Geometry check sheet. Reference: the model listing, model coordinates, mm. Coordinates: 2 decimals unless noted, no trailing zeros. Order: outer loops, then holes, each group sorted by start corner. A loop starts at its lowest first (then second) coordinate and runs counter-clockwise, first axis right, second up. Notation, with made-up numbers: M 69,-22.75 L 97,-22.75 A10 ccw 97,-8.75 Z; hole C 75,-39 d6. An arc over 180 degrees is marked long. One line per item, written item: value. Start each with the question number.
1) Sectioned sample at A-A, the plane x = 26. Enter the section's corners in (y, z) (3 decimals).
2) Sectioned sample at D-D, the plane x = 145. Enter the section's corners in (y, z) (3 decimals).
3) Sectioned sample at C-C, the plane y = 1.75. State how many separate pieces and enclosed holes the cut face has, then the cut area to 3 significant figures.
4) Thickness scan on L1, parallel to Z at x = 151, y = 2.2; L2, parallel to Z at x = 104.5, y = 0.5 (3 decimals); L3, parallel to X at y = 3, z = -44. Record the ranges inside material, lowest first. Write a range as from..to.
5) Go/stop test with a flat-tipped pin: P1, Ø2.5, axis at x = 4, z = -4, coming from the +Y side. Record where the tip stops, or that it passes through.
6) Draft check along X on faces 1 (the flat face through (0, 1, -35)), 2 (the flat face through (82, 0, -25)), 3 (the flat face through (155, 1, -35)). Enter one of: pulls with the +X half, pulls with the -X half, needs draft (parallel to the pull), parting line crosses it, or undercut.
```python
from build123d import *

# Parameters (mm, degrees)
SKETCH1_R           = 1.5
SKETCH1_W           = 19.05
SKETCH1_H           = 19.05
BOSS_EXTRUDE1_DEPTH = 3.75
SKETCH2_W           = 9.525
SKETCH2_H           = 3.75
BOSS_EXTRUDE2_DEPTH = 20
SKETCH3_W           = 17.05
SKETCH3_H           = 3.75
CUT_EXTRUDE1_DEPTH  = 2
SKETCH4_W           = 88.15
SKETCH4_H           = 3.75
BOSS_EXTRUDE3_DEPTH = 4
SKETCH5_W           = 13.325
SKETCH5_H           = 3.75
BOSS_EXTRUDE4_DEPTH = 6
SKETCH6_W           = 19.675
SKETCH6_H           = 3.75
BOSS_EXTRUDE5_DEPTH = 10
SKETCH7_W           = 11
SKETCH7_H           = 3.75
CUT_EXTRUDE2_DEPTH  = 4
SKETCH8_W           = 33
SKETCH8_H           = 3.75
BOSS_EXTRUDE6_DEPTH = 1.0375
SKETCH9_W           = 38.1
SKETCH9_H           = 3.75
CUT_EXTRUDE3_DEPTH  = 0.5
SKETCH10_W          = 52.725
SKETCH10_H          = 3.75
CUT_EXTRUDE4_DEPTH  = 0.5
SKETCH11_W          = 18
SKETCH11_H          = 3.75
CUT_EXTRUDE5_DEPTH  = 0.5
SKETCH13_W          = 14.7
SKETCH13_H          = 3.75
CUT_EXTRUDE6_DEPTH  = 2.175
FILLET1_R           = 0.5
BOSS_EXTRUDE7_START = 3
BOSS_EXTRUDE7_DEPTH = 3
FILLET2_R           = 0.5
FILLET3_R           = 0.5


with BuildPart() as part:
    # Sketch1 → Boss-Extrude1 (new body)
    with BuildSketch(Plane(origin=(0, 0, 0), x_dir=(1, 0, 0), z_dir=(0, 1, 0))):
        with BuildLine():
            ThreePointArc((0, 0.5), (0.146446609, 0.146446609), (0.5, 0))
            Line((0.5, 0), (154.5, 0))
            ThreePointArc((154.5, 0), (154.853553391, 0.146446609), (155, 0.5))
            Line((155, 0.5), (155, 69.5))
            ThreePointArc((155, 69.5), (154.853553391, 69.853553391), (154.5, 70))
            Line((154.5, 70), (132.3125, 70))
            Line((132.3125, 70), (132.3125, 63.825))
            Line((132.3125, 63.825), (146.5125, 63.825))
            Line((146.5125, 63.825), (146.5125, 46.325))
            Line((146.5125, 46.325), (132.3125, 46.325))
            Line((132.3125, 46.325), (91.7875, 46.325))
            Line((91.7875, 46.325), (89.7875, 46.325))
            Line((89.7875, 46.325), (89.7875, 35))
            Line((89.7875, 35), (72.7375, 35))
            Line((72.7375, 35), (72.7375, 15.95))
            Line((72.7375, 15.95), (53.6875, 15.95))
            Line((53.6875, 15.95), (53.6875, 35))
            Line((53.6875, 35), (44.1625, 35))
            Line((44.1625, 35), (44.1625, 6.425))
            Line((44.1625, 6.425), (6.0625, 6.425))
            Line((6.0625, 6.425), (6.0625, 63.575))
            Line((6.0625, 63.575), (44.1625, 63.575))
            Line((44.1625, 63.575), (44.1625, 70))
            Line((44.1625, 70), (0.5, 70))
            ThreePointArc((0.5, 70), (0.146446609, 69.853553391), (0, 69.5))
            Line((0, 69.5), (0, 0.5))
        make_face()
        with Locations(Location((4, 4, 0), (0, 0, 270))):
            Circle(SKETCH1_R, mode=Mode.SUBTRACT)
        with Locations(Location((151, 4, 0), (0, 0, 270))):
            Circle(SKETCH1_R, mode=Mode.SUBTRACT)
        with Locations(Location((82.2625, 25.475, 0), (0, 0, 270))):
            Circle(SKETCH1_R, mode=Mode.SUBTRACT)
        with Locations((101.3125, 25.475)):
            Rectangle(SKETCH1_W, SKETCH1_H, mode=Mode.SUBTRACT)
        with Locations(Location((120.3625, 25.475, 0), (0, 0, 270))):
            Circle(SKETCH1_R, mode=Mode.SUBTRACT)
        with Locations((139.4125, 25.475)):
            Rectangle(SKETCH1_W, SKETCH1_H, mode=Mode.SUBTRACT)
        with Locations(Location((4, 66, 0), (0, 0, 270))):
            Circle(SKETCH1_R, mode=Mode.SUBTRACT)
        with Locations(Location((151, 66, 0), (0, 0, 270))):
            Circle(SKETCH1_R, mode=Mode.SUBTRACT)
    extrude(amount=BOSS_EXTRUDE1_DEPTH)

    # Sketch2 → Boss-Extrude2 (add)
    with BuildSketch(Plane(origin=(0, 0, -35), x_dir=(-1, 0, 0), z_dir=(0, 0, -1))):
        with Locations((-48.925, 1.875)):
            Rectangle(SKETCH2_W, SKETCH2_H)
    extrude(amount=BOSS_EXTRUDE2_DEPTH)

    # Sketch3 → Cut-Extrude1 (cut)
    with BuildSketch(Plane(origin=(0, 0, -35), x_dir=(-1, 0, 0), z_dir=(0, 0, -1))):
        with Locations((-81.2625, 1.875)):
            Rectangle(SKETCH3_W, SKETCH3_H)
    extrude(amount=-CUT_EXTRUDE1_DEPTH, mode=Mode.SUBTRACT)

    # Sketch4 → Boss-Extrude3 (add)
    with BuildSketch(Plane(origin=(0, 0, -70), x_dir=(-1, 0, 0), z_dir=(0, 0, -1))):
        with Locations((-88.2375, 1.875)):
            Rectangle(SKETCH4_W, SKETCH4_H)
    extrude(amount=-BOSS_EXTRUDE3_DEPTH)

    # Sketch5 → Boss-Extrude4 (add)
    with BuildSketch(Plane.ZY.offset(-89.7875)):
        with Locations((-39.6625, 1.875)):
            Rectangle(SKETCH5_W, SKETCH5_H)
    extrude(amount=BOSS_EXTRUDE4_DEPTH)

    # Sketch6 → Boss-Extrude5 (add)
    with BuildSketch(Plane.ZY.offset(-83.7875)):
        with Locations((-56.1625, 1.875)):
            Rectangle(SKETCH6_W, SKETCH6_H)
    extrude(amount=-BOSS_EXTRUDE5_DEPTH)

    # Sketch7 → Cut-Extrude2 (cut)
    with BuildSketch(Plane(origin=(0, 0, -70), x_dir=(-1, 0, 0), z_dir=(0, 0, -1))):
        with Locations((-77.25, 1.875)):
            Rectangle(SKETCH7_W, SKETCH7_H)
    extrude(amount=-CUT_EXTRUDE2_DEPTH, mode=Mode.SUBTRACT)

    # Sketch8 → Boss-Extrude6 (add)
    with BuildSketch(Plane.ZY.offset(-83.7875)):
        with Locations((-49.5, 1.875)):
            Rectangle(SKETCH8_W, SKETCH8_H)
    extrude(amount=BOSS_EXTRUDE6_DEPTH)

    # Sketch9 → Cut-Extrude3 (cut)
    with BuildSketch(Plane(origin=(0, 0, -6.425), x_dir=(-1, 0, 0), z_dir=(0, 0, -1))):
        with Locations((-25.1125, 1.875)):
            Rectangle(SKETCH9_W, SKETCH9_H)
    extrude(amount=-CUT_EXTRUDE3_DEPTH, mode=Mode.SUBTRACT)

    # Sketch10 → Cut-Extrude4 (cut)
    with BuildSketch(Plane(origin=(0, 0, -46.325), x_dir=(-1, 0, 0), z_dir=(0, 0, -1))):
        with Locations((-120.15, 1.875)):
            Rectangle(SKETCH10_W, SKETCH10_H)
    extrude(amount=-CUT_EXTRUDE4_DEPTH, mode=Mode.SUBTRACT)

    # Sketch11 → Cut-Extrude5 (cut)
    with BuildSketch(Plane.ZY.offset(-146.5125)):
        with Locations((-54.825, 1.875)):
            Rectangle(SKETCH11_W, SKETCH11_H)
    extrude(amount=-CUT_EXTRUDE5_DEPTH, mode=Mode.SUBTRACT)

    # Sketch13 → Cut-Extrude6 (cut)
    with BuildSketch(Plane.XY.offset(-63.825)):
        with Locations((139.6625, 1.875)):
            Rectangle(SKETCH13_W, SKETCH13_H)
    extrude(amount=-CUT_EXTRUDE6_DEPTH, mode=Mode.SUBTRACT)

    # Fillet1
    fillet1_edges = [part.edges().sort_by_distance(p)[0] for p in [
        (72.7375, 1.875, -33),
        (129.8875, 1.875, -35),
        (91.7875, 1.875, -35),
        (44.1625, 1.875, -66),
        (93.7875, 1.875, -66),
        (71.75, 1.875, -66),
        (82.75, 1.875, -33),
        (44.1625, 1.875, -5.925),
        (6.0625, 1.875, -5.925),
        (93.7875, 1.875, -45.825),
        (147.0125, 1.875, -45.825),
        (147.0125, 1.875, -66),
        (72.7375, 1.875, -15.95),
        (53.6875, 1.875, -15.95),
        (6.0625, 1.875, -63.575),
        (148.9375, 1.875, -35),
        (148.9375, 1.875, -15.95),
        (129.8875, 1.875, -15.95),
        (53.6875, 1.875, -55),
        (44.1625, 1.875, -55),
        (110.8375, 1.875, -35),
        (110.8375, 1.875, -15.95),
        (91.7875, 1.875, -15.95),
        (44.1625, 1.875, -63.575),
    ]]
    fillet(fillet1_edges, radius=FILLET1_R)

    # Sketch12 → Boss-Extrude7 (add)
    with BuildSketch(Plane.XZ.offset(BOSS_EXTRUDE7_START)):
        with BuildLine():
            Line((155, -0.5), (155, -69.5))
            ThreePointArc((155, -69.5), (154.853553391, -69.853553391), (154.5, -70))
            Line((154.5, -70), (0.5, -70))
            ThreePointArc((0.5, -70), (0.146446609, -69.853553391), (0, -69.5))
            Line((0, -69.5), (0, -0.5))
            ThreePointArc((0, -0.5), (0.146446609, -0.146446609), (0.5, 0))
            Line((0.5, 0), (154.5, 0))
            ThreePointArc((154.5, 0), (154.853553391, -0.146446609), (155, -0.5))
        make_face()
    extrude(amount=-BOSS_EXTRUDE7_DEPTH)

    # Fillet2
    fillet2_edges = [part.edges().sort_by_distance(p)[0] for p in [
        (154.853553391, -3, -0.146446609),
        (77.5, -3, 0),
        (0.146446609, -3, -0.146446609),
        (0, -3, -35),
        (0.146446609, -3, -69.853553391),
        (77.5, -3, -70),
        (154.853553391, -3, -69.853553391),
        (155, -3, -35),
    ]]
    fillet(fillet2_edges, radius=FILLET2_R)

    # Fillet3
    fillet3_edges = [part.edges().sort_by_distance(p)[0] for p in [
        (147.0125, 0, -55.9125),
        (120.4, 0, -66),
        (120.4, 0, -45.825),
        (53.6875, 0, -35.475),
        (63.2125, 0, -15.95),
        (25.1125, 0, -5.925),
        (44.1625, 0, -30.4625),
        (6.0625, 0, -34.75),
        (25.1125, 0, -63.575),
        (48.925, 0, -55),
        (93.7875, 0, -55.9125),
        (72.7375, 0, -24.475),
        (77.74375, 0, -33),
        (82.75, 0, -51.75),
        (71.75, 0, -68.25),
        (57.95625, 0, -66),
        (44.1625, 0, -64.7875),
        (110.8375, 0, -25.475),
        (101.3125, 0, -35),
        (91.7875, 0, -25.475),
        (101.3125, 0, -15.95),
        (148.9375, 0, -25.475),
        (139.4125, 0, -35),
        (129.8875, 0, -25.475),
        (139.4125, 0, -15.95),
        (72.883946609, 0, -32.853553391),
        (71.603553391, 0, -66.146446609),
        (44.016053391, 0, -63.721446609),
        (53.541053391, 0, -54.853553391),
        (44.308946609, 0, -54.853553391),
        (146.866053391, 0, -65.853553391),
        (146.866053391, 0, -45.971446609),
        (53.833946609, 0, -16.096446609),
        (44.016053391, 0, -6.071446609),
        (6.208946609, 0, -6.071446609),
        (6.208946609, 0, -63.428553391),
        (44.308946609, 0, -65.853553391),
        (72.591053391, 0, -16.096446609),
        (82.603553391, 0, -33.146446609),
        (93.933946609, 0, -65.853553391),
        (93.933946609, 0, -45.971446609),
        (91.933946609, 0, -16.096446609),
        (91.933946609, 0, -34.853553391),
        (110.691053391, 0, -16.096446609),
        (110.691053391, 0, -34.853553391),
        (130.033946609, 0, -16.096446609),
        (130.033946609, 0, -34.853553391),
        (148.791053391, 0, -34.853553391),
        (148.791053391, 0, -16.096446609),
    ]]
    fillet(fillet3_edges, radius=FILLET3_R)


solid = part.part
```
Final values:
1. outline: M -3,-69.5 A0.5 ccw -2.5,-70 L 3.75,-70 L 3.75,-63.575 L 0.5,-63.575 A0.5 cw 0,-63.075 L 0,-6.425 A0.5 cw 0.5,-5.925 L 3.75,-5.925 L 3.75,0 L -2.5,0 A0.5 ccw -3,-0.5 Z
2. outline: M -3,-69.5 A0.5 ccw -2.5,-70 L 3.75,-70 L 3.75,-66 L 0.5,-66 A0.5 cw 0,-65.5 L 0,-46.325 A0.5 cw 0.5,-45.825 L 3.75,-45.825 L 3.75,-35 L 0.5,-35 A0.5 cw 0,-34.5 L 0,-16.45 A0.5 cw 0.5,-15.95 L 3.75,-15.95 L 3.75,0 L -2.5,0 A0.5 ccw -3,-0.5 Z
3. separate pieces: 1
3. enclosed holes: 9
3. area: 5,380 mm^2
4. L1: z = -70..-67.5, -64.5..-5.5, -2.5..0
4. L2: z = -70..-66, -45.825..-35, -15.95..0
4. L3: x = 0..6.06, 44.16..53.69, 82.75..155
5. P1: stops at y = 0
6. face 1: pulls with the -X half
6. face 2: undercut
6. face 3: pulls with the +X half
